For this review, take the finished solid that the model builds, in its own axes (mm). Face numbers are marked on the shaded views. A direction names the side the tool comes from. Give positions to 0.01 mm unless a question says otherwise; leave off trailing zeros. Order: outer loops, then holes, each group sorted by start corner. A loop starts at its lowest first (then second) coordinate and runs counter-clockwise, first axis right, second up. Notation, with made-up numbers: M -31,16.25 L 6,16.25 A19 cw 6,48.25 Z; hole C 48.5,68.5 d11. An arc over 180 degrees is marked long. Use CSV: the item, a comma, the result in double quotes. Start each with the question number.
(1) Consider section B-B (x = -7.75). Write out the cut boundary in (y, z).
(2) Tool access review of the marked faces 1, 2 and 3: name each direction out of +Z, -Z, +X, -X, +Y, -Y from which nothing blocks a thin tool from reaching the whole face with its end or side.
(3) Clearance check with flat-ended pins moving along their axes: P1, Ø1, axis at x = 1, z = 1.5, coming from the -Y side; P2, Ø1.9, axis at y = 18.85, z = -22.98, coming from the +X side; P3, Ø3.5, axis at x = 0, z = -27.5, coming from the +Y side; P4, Ø5, axis at x = -2, z = -10, coming from the +Y side. State where each tip first meets the part, or that it passes through.
(4) Consider section D-D (x = 3). Write out the cut boundary in (y, z), and give its area (3 significant figures).
(5) Consider section A-A (x = -2.25). Write out the cut boundary in (y, z).
(6) Draft analysis for pull direction Y (two halves, no side actions). For the marked faces 4, 5 and 6, state which applies: pulls with the +Y half, pulls with the -Y half, needs draft (parallel to the pull), parting line crosses it, or undercut.
(7) Wall thickness on L1, parallel to Y at x = 3.5, z = 2; L2, parallel to Y at x = 1.5, z = 23; L3, parallel to X at y = 41, z = 15: over which ranges is each line inside the solid? List them lowest first. Write a range as from..to.
(8) Consider section C-C (z = 0). Give the number of separate pieces and of enclosed holes in the cut face, and give its area (3 significant figures).
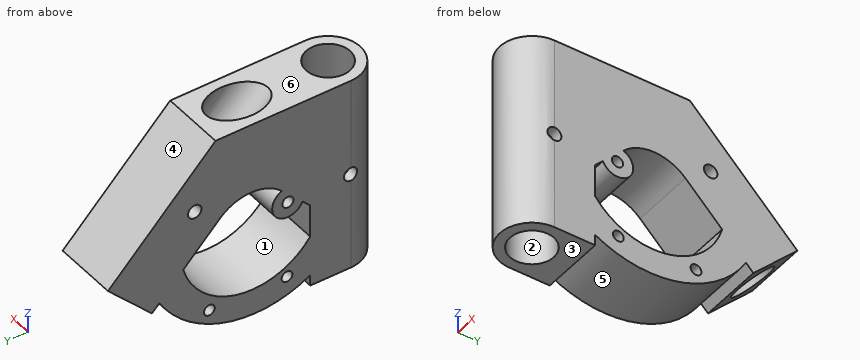
```python
from build123d import *

# Parameters (mm, degrees)
CROQUIS1_R              = 6.5
SALIENTE_EXTRUIR1_DEPTH = 29
SALIENTE_EXTRUIR2_DEPTH = 9.5
CROQUIS3_R              = 6.5
CORTAR_EXTRUIR1_DEPTH   = 73
SALIENTE_EXTRUIR3_DEPTH = 9.5
CROQUIS5_R              = 4.65
CROQUIS5_R_2            = 1.65
SALIENTE_EXTRUIR4_DEPTH = 9.5
CROQUIS6_R              = 1.6
CORTAR_EXTRUIR2_DEPTH   = 15
CROQUIS7_R              = 2
CORTAR_EXTRUIR3_DEPTH   = 26.5


with BuildPart() as part:
    # Croquis1 → Saliente-Extruir1 (new body, symmetric)
    with BuildSketch(Plane.XY):
        with BuildLine():
            Line((-9.5, 12), (9.5, 12))
            Line((9.5, 12), (9.5, 0))
            ThreePointArc((9.5, 0), (0, -9.5), (-9.5, 0))
            Line((-9.5, 0), (-9.5, 12))
        make_face()
        Circle(CROQUIS1_R, mode=Mode.SUBTRACT)
    extrude(amount=SALIENTE_EXTRUIR1_DEPTH, both=True)

    # Croquis2 → Saliente-Extruir2 (add, symmetric)
    with BuildSketch(Plane(origin=(0, 0, 0), x_dir=(0, 0, -1), z_dir=(1, 0, 0))):
        with BuildLine():
            Line((-29, 12), (-29, 40))
            Line((-29, 40), (2.819805153, 71.819805153))
            Line((2.819805153, 71.819805153), (15.830569927, 58.80904038))
            Line((15.830569927, 58.80904038), (-4.251796904, 38.726673548))
            ThreePointArc((-4.251796904, 38.726673548), (-8.059408749, 29.534285393), (-4.251796904, 20.341897237))
            Line((-4.251796904, 20.341897237), (4.090100333, 12))
            Line((4.090100333, 12), (-29, 12))
        make_face()
    extrude(amount=SALIENTE_EXTRUIR2_DEPTH, both=True)

    # Croquis3 → Cortar-Extruir1 (cut)
    with BuildSketch(Plane(origin=(0, 37.319805153, -37.319805153), x_dir=(1, 0, 0), z_dir=(0, 0.707106781, -0.707106781))):
        with Locations((0, -39.590367902)):
            Circle(CROQUIS3_R)
    extrude(amount=-CORTAR_EXTRUIR1_DEPTH, mode=Mode.SUBTRACT)

    # Croquis4 → Saliente-Extruir3 (add, symmetric)
    with BuildSketch(Plane(origin=(0, 0, 0), x_dir=(0, 0, -1), z_dir=(1, 0, 0))):
        with BuildLine():
            Line((6.58232419, 49.560794642), (13.653392001, 56.631862454))
            ThreePointArc((13.653392001, 56.631862454), (28.845023505, 36.796295198), (25.782485256, 12))
            Line((25.782485256, 12), (13.782485256, 12))
            ThreePointArc((13.782485256, 12), (21.90502045, 33.027546833), (6.58232419, 49.560794642))
        make_face()
    extrude(amount=SALIENTE_EXTRUIR3_DEPTH, both=True)

    # Croquis5 → Saliente-Extruir4 (add, symmetric)
    with BuildSketch(Plane(origin=(0, 0, 0), x_dir=(0, 0, -1), z_dir=(1, 0, 0))):
        with Locations((0, 18.59255238)):
            Circle(CROQUIS5_R)
        with Locations((0, 18.59255238)):
            Circle(CROQUIS5_R_2, mode=Mode.SUBTRACT)
    extrude(amount=SALIENTE_EXTRUIR4_DEPTH, both=True)

    # Croquis6 → Cortar-Extruir2 (cut, symmetric)
    with BuildSketch(Plane(origin=(0, 0, 0), x_dir=(0, 0, -1), z_dir=(1, 0, 0))):
        with Locations((22.726275042, 41.82542613)):
            Circle(CROQUIS6_R)
        with Locations((22.98, 18.84542613)):
            Circle(CROQUIS6_R)
    extrude(amount=CORTAR_EXTRUIR2_DEPTH, both=True, mode=Mode.SUBTRACT)

    # Croquis7 → Cortar-Extruir3 (cut, symmetric)
    with BuildSketch(Plane(origin=(0, 0, 0), x_dir=(0, 0, -1), z_dir=(1, 0, 0))):
        Circle(CROQUIS7_R)
        with Locations((-9.83740623, 46.151828996)):
            Circle(CROQUIS7_R)
    extrude(amount=CORTAR_EXTRUIR3_DEPTH, both=True, mode=Mode.SUBTRACT)


solid = part.part
```
Check result:
1,outline,"M -5.49,-29 L 12,-29 L 12,-25.78 A33 ccw 56.63,-13.65 L 58.81,-15.83 L 71.82,-2.82 L 40,29 L -5.49,29 Z; hole C 0,0 d4; hole M 12,-13.78 A21.29 ccw 49.56,-6.58 L 38.73,4.25 A13 ccw 20.38,4.29 A4.65 cw long 14.3,-1.79 L 12,-4.09 Z; hole C 18.59,0 d3.3; hole C 18.85,-22.98 d3.2; hole C 41.83,-22.73 d3.2; hole C 46.15,9.84 d4"
2,face 1,"+X, -X"
2,face 2,"+Z, -Z"
2,face 3,"-Z, +X, -X, -Y"
3,P1,"stops at y = -9.49"
3,P2,"passes through"
3,P3,"stops at y = 44.34"
3,P4,"stops at y = 60.27"
4,outline,"M -9.01,-29 L -5.77,-29 L -5.77,29 L -9.01,29 Z; M 5.77,-29 L 12,-29 L 12,-25.78 A33 ccw 56.63,-13.65 L 58.81,-15.83 L 61.24,-13.4 L 18.83,29 L 5.77,29 Z; M 35.14,29 L 69.39,-5.25 L 71.82,-2.82 L 40,29 Z; hole M 12,-13.78 A21.29 ccw 49.56,-6.58 L 38.73,4.25 A13 ccw 20.38,4.29 A4.65 cw long 14.3,-1.79 L 12,-4.09 Z; hole C 18.59,0 d3.3; hole C 18.85,-22.98 d3.2; hole C 41.83,-22.73 d3.2"
4,area,"1,690 mm^2"
5,outline,"M -9.23,-29 L -6.1,-29 L -6.1,29 L -9.23,29 Z; M 6.1,-29 L 12,-29 L 12,-25.78 A33 ccw 56.63,-13.65 L 58.81,-15.83 L 61,-13.64 L 18.37,29 L 6.1,29 Z; M 35.61,29 L 69.63,-5.01 L 71.82,-2.82 L 40,29 Z; hole M 12,-13.78 A21.29 ccw 49.56,-6.58 L 38.73,4.25 A13 ccw 20.38,4.29 A4.65 cw long 14.3,-1.79 L 12,-4.09 Z; hole C 18.59,0 d3.3; hole C 18.85,-22.98 d3.2; hole C 41.83,-22.73 d3.2"
6,face 4,"pulls with the +Y half"
6,face 5,"undercut"
6,face 6,"needs draft"
7,L1,"y = -8.83..-5.48, 5.48..22.79, 40.98..46.24, 61.74..67"
7,L2,"y = -9.38..-6.32, 6.32..24.04, 41.93..46"
7,L3,"x = -9.5..-6.5, 6.5..9.5"
8,separate pieces,"4"
8,enclosed holes,"1"
8,area,"670 mm^2"
